For this review, use the dimensioned drawing (mm, ordinates from the lowest corner) and the shaded views. A direction names the side the tool comes from. Round coordinates to 2 decimals unless told otherwise and drop trailing zeros. Write each loop counter-clockwise with the first axis right and the second up, starting at its lowest first coordinate (ties: lowest second). Pieces come first, ordered by that corner, then holes. Notation, with made-up numbers: M 13.5,-5 L 24.5,-5 A11 cw 24.5,9 Z; hole C 14,-18.5 d6. An arc over 180 degrees is marked long. One line per question, with ' | ' between items.
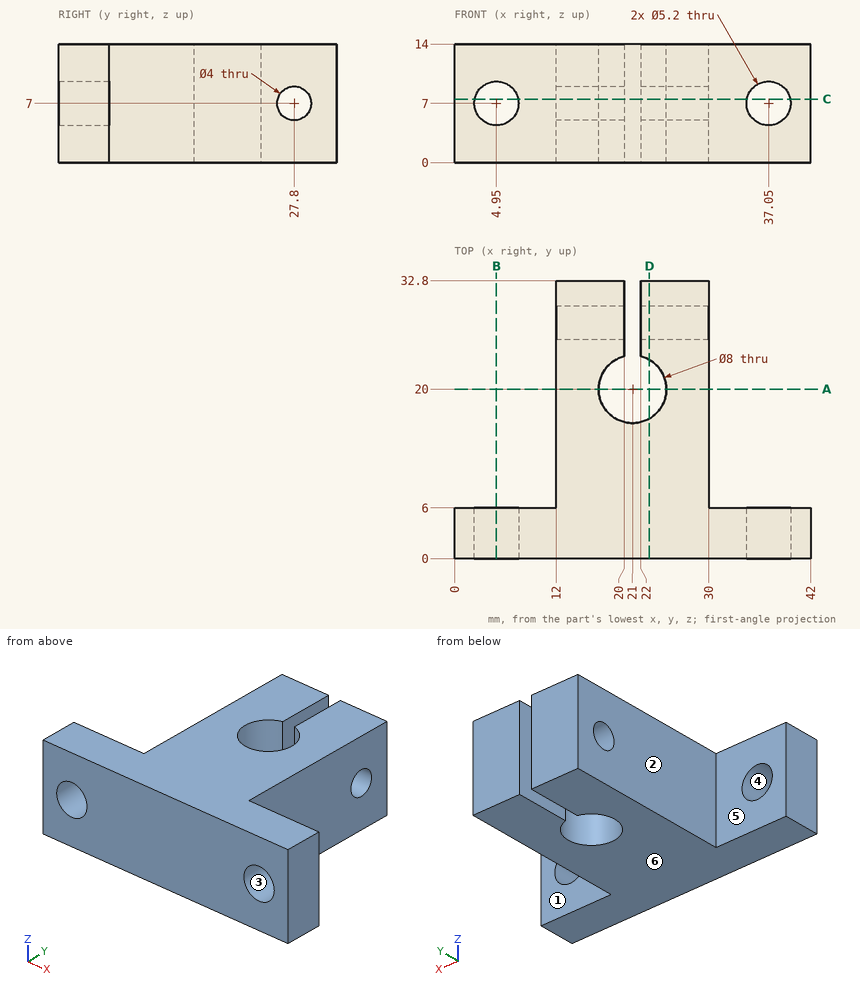
Item 1: Insertion check: pin 1 Ø4 at (x, z) = (4.95, 7) entering from +Y; pin 2 Ø8 at (y, z) = (29, 1.5) entering from +X; pin 3 Ø6 at (x, z) = (33.5, 9) entering from +Y. Each pin has a flat end and moves straight along its axis. Give the tip position at first contact, or say it passes through.
Results:
pin 1: through | pin 2: x = 30 | pin 3: y = 6
Item 2: To check wall thickness, follow line 1 along X through (y, z) = (30.5, 4.75); line 2 along X through (y, z) = (4, 7); line 3 along Y through (x, z) = (25.5, 7). State the ranges of each line that lie inside material, in increasing order. Write a range as from..to.
Results:
line 1: 12..20, 22..30 | line 2: 0..2.35, 7.55..34.45, 39.65..42 | line 3: 0..25.8, 29.8..32.8
Item 3: Take a section at A-A (y = 20). Write out the cut boundary in (x, z), then the cut area to 3 significant figures.
Results:
outline: M 12,0 L 17,0 L 17,14 L 12,14 Z; M 25,0 L 30,0 L 30,14 L 25,14 Z | area: 140 mm2
Item 4: Take a section at B-B (x = 4.95). Write out the cut boundary in (y, z).
Results:
outline: M 0,0 L 6,0 L 6,4.4 L 0,4.4 Z; M 0,9.6 L 6,9.6 L 6,14 L 0,14 Z
Item 5: Take a section at C-C (z = 7.5). Write out the cut boundary in (x, y).
Results:
outline: M 0,0 L 2.4,0 L 2.4,6 L 0,6 Z; M 7.5,0 L 34.5,0 L 34.5,6 L 30,6 L 30,25.86 L 22,25.86 L 22,23.87 A4 cw long 20,23.87 L 20,25.86 L 12,25.86 L 12,6 L 7.5,6 Z; M 12,29.74 L 20,29.74 L 20,32.8 L 12,32.8 Z; M 22,29.74 L 30,29.74 L 30,32.8 L 22,32.8 Z; M 39.6,0 L 42,0 L 42,6 L 39.6,6 Z
Item 6: Take a section at D-D (x = 23). Write out the cut boundary in (y, z).
Results:
outline: M 0,0 L 16.54,0 L 16.54,14 L 0,14 Z; M 23.46,0 L 32.8,0 L 32.8,14 L 23.46,14 Z; hole C 27.8,7 d4
Item 7: Machinability: for the marked faces 1, 2 and 3, which of the approach directions +Z, -Z, +X, -X, +Y, -Y give a long, thin tool a straight path to every point of the face, cutting with its end or side? Answer none if there is none.
Results:
face 1: +Z, -Z, +X, +Y | face 2: +Z, -Z, -X, +Y | face 3: +Y, -Y
Item 8: Mouldability with a two-part tool opening along Z and no side actions: class the marked faces 4, 5 and 6 as +Z half, -Z half, draft (parallel to the pull), parting line (faces both ways), or undercut.
Results:
face 4: undercut | face 5: draft | face 6: -Z half
